from build123d import *

# Parameters (mm, degrees)
F0_R     = 27.686
F1_DEPTH = 6.35
F2_D     = 18.288
F3_R     = 31.75
F5_DEPTH = 26.67
F5_TAPER = 30
F7_D     = 18.288


with BuildPart() as f1:
    # F0 (on Top) → F1 (new body)
    with BuildSketch(Plane.XY):
        Circle(F0_R)
    extrude(amount=F1_DEPTH)

    # F2 (through all)
    with Locations(Plane(origin=(0, 0, 0), x_dir=(1, 0, 0), z_dir=(0, 0, -1))):
        with Locations((0, 0)):
            Hole(F2_D / 2)

    # F3 (on Top) → F5 (join)
    with BuildSketch(Plane.XY):
        Circle(F3_R)
    extrude(amount=-F5_DEPTH, taper=F5_TAPER)

    # F7 (through all)
    with Locations(Plane(origin=(0, 0, -26.67), x_dir=(1, 0, 0), z_dir=(0, 0, -1))):
        with Locations((0, 0)):
            Hole(F7_D / 2)


solid = f1.part
Work out the finished part from the listing and answer in its coordinate system (mm). A direction names the side the tool comes from. Coordinates: 2 decimals unless noted, no trailing zeros. Write each loop counter-clockwise with the first axis right and the second up, starting at its lowest first coordinate (ties: lowest second). Pieces come first, ordered by that corner, then holes.
1. The part is cut by section C-C, the plane z = -18. Write down the section's boundary in (x, y), and give its area (3 significant figures).
Results list:
outline: circle Ø42.72 at (0, 0); hole circle Ø18.29 at (0, 0)
area: 1,170 mm2
2. The part is cut by section A-A, the plane x = 0. Write down the section's boundary in (y, z), and give its area (3 significant figures).
Results list:
outline: (-31.75, 0) - (-16.35, -26.67) - (-9.14, -26.67) - (-9.14, 6.35) - (-27.69, 6.35) - (-27.69, 0) - close; (9.14, -26.67) - (16.35, -26.67) - (31.75, 0) - (27.69, 0) - (27.69, 6.35) - (9.14, 6.35) - close
area: 1,030 mm2
3. The part is cut by section B-B, the plane z = -22.5. Write down the section's boundary in (x, y), and give its area (3 significant figures).
Results list:
outline: circle Ø37.52 at (0, 0); hole circle Ø18.29 at (0, 0)
area: 843 mm2
4. For a pull along Y with two mould halves and no side action, classify faces 3 (the flat face through (-10, 26, 0)), 4 (the conical face through (-4.078, -18.363, -22.412)), 5 (the cylindrical face through (1.982, 8.927, -9.929)) as +Y half, -Y half, draft (parallel to the pull), parting line (faces both ways), or undercut.
Results list:
face 3: draft
face 4: parting line
face 5: undercut
5. For faces 1 (the cylindrical face through (14.884, 23.345, 3.131)), 2 (the flat face through (7, -7, -26.67)), determine the directions among +Z, -Z, +X, -X, +Y, -Y from which every point of the face is accessible in a straight line to the end or side of a thin tool.
Results list:
face 1: +Z
face 2: -Z, +X, -X, +Y, -Y
6. Flat-ended cylindrical pins translate along their axes: pin 1 (10 mm diameter, centred on x = 19, z = -22, fed in from -Y); pin 2 (2 mm diameter, centred on x = -8.5, y = -19.5, fed in from -Z); pin 3 (3 mm diameter, centred on x = 6.5, z = -0.5, fed in from +Y). Find the tip coordinate at first contact, or state that the pin passes through.
Results list:
pin 1: stops at y = -14.38
pin 2: stops at z = -19.88
pin 3: stops at y = 31.34
7. Consider line 1 along X through (y, z) = (-1.5, -20.5); line 2 along Y through (x, z) = (0, -17.5); line 3 along Y through (x, z) = (0, -20). Determine where each line is inside the solid, lowest interval first.
Results list:
line 1: x = -19.86 to -9.02, 9.02 to 19.86
line 2: y = -21.65 to -9.14, 9.14 to 21.65
line 3: y = -20.2 to -9.14, 9.14 to 20.2
